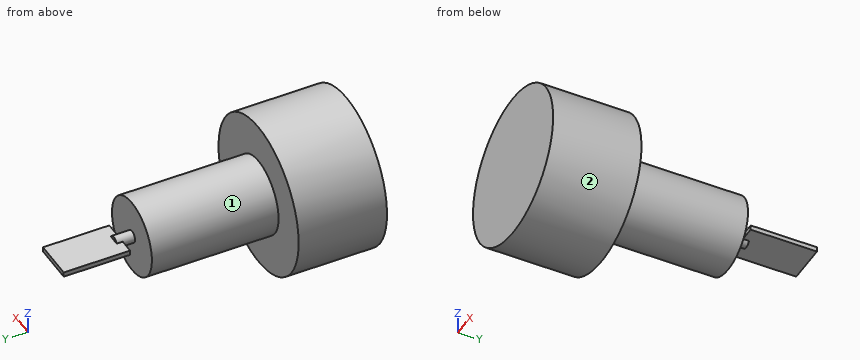
```python
from build123d import *

# Parameters (mm, degrees)
SKETCH_1_R           = 12.75
EXTRUDE_1_DEPTH      = 14.65
SKETCH_2_R           = 6.35
EXTRUDE_2_DEPTH      = 21
SKETCH_3_R           = 1
EXTRUDE_3_DEPTH      = 3
EXTRUDE_4_DEPTH      = 0.4
EXTRUDE_4_DEPTH_BACK = 0.4
SKETCH_4_W           = 6.6
SKETCH_4_H           = 11


with BuildPart() as part:
    # Sketch 1 → Extrude 1 (new body)
    with BuildSketch(Plane(origin=(0, 0, 0), x_dir=(1, 0, 0), z_dir=(0, 1, 0))):
        with Locations(Location((0, 0, 0), (0, 0, 270))):
            Circle(SKETCH_1_R)
    extrude(amount=EXTRUDE_1_DEPTH)

    # Sketch 2 → Extrude 2 (add)
    with BuildSketch(Plane(origin=(0, 14.65, 0), x_dir=(1, 0, 0), z_dir=(0, 1, 0))):
        with Locations(Location((0, 0, 0), (0, 0, 90))):
            Circle(SKETCH_2_R)
    extrude(amount=EXTRUDE_2_DEPTH)

    # Sketch 3 → Extrude 3 (add)
    with BuildSketch(Plane(origin=(0, 35.65, 0), x_dir=(1, 0, 0), z_dir=(0, 1, 0))):
        with Locations(Location((0, 0, 0), (0, 0, 270))):
            Circle(SKETCH_3_R)
    extrude(amount=EXTRUDE_3_DEPTH)

    # Sketch 4 → Extrude 4 (add, two sides: drawn at the far end of the back side and taken through both)
    with BuildSketch(Plane.XY.offset(-EXTRUDE_4_DEPTH_BACK)):
        with Locations((0.05, 43.15)):
            Rectangle(SKETCH_4_W, SKETCH_4_H)
    extrude(amount=EXTRUDE_4_DEPTH + EXTRUDE_4_DEPTH_BACK)


solid = part.part
```
The listing builds one solid part. Answer for the finished solid, in the listing's coordinates (mm). Face numbers are marked on the shaded views. A direction names the side the tool comes from. Round coordinates to 2 decimals unless told otherwise and drop trailing zeros. Loops run counter-clockwise (first coordinate to the right, second up) from the corner with the lowest first, then second, coordinate; pieces in that order, holes last.
Q1. Section C-C, the plane z = -7.25 is taken. Determine the outline of the cut face in (x, y).
Q2. Section A-A, the plane x = 0 is taken. Determine the outline of the cut face in (y, z), then the cut area to 3 significant figures.
Q3. Given pin 1 Ø10 at (x, y) = (8, 39.5) entering from -Z; pin 2 Ø4 at (x, y) = (3, 19.5) entering from -Z; pin 3 Ø8 at (x, y) = (-7, 12) entering from -Z, each flat-ended and moving along its own axis, determine where each tip first touches the part or whether it passes through.
Q4. Section B-B, the plane y = 20 is taken. Determine the outline of the cut face in (x, z), then the cut area to 3 significant figures.
Q5. Which of the six approach directions +Z, -Z, +X, -X, +Y, -Y give full straight-line access (tool end or side, diameter ignored) to the marked faces 1 and 2?
Q6. Section D-D, the plane y = 8 is taken. Determine the outline of the cut face in (x, z), then the cut area to 3 significant figures.
Q7. Find the intervals of material crossed by line 1 (Y direction, x = -4, z = -7.25); line 2 (Y direction, x = -5.25, z = -1.75); line 3 (Z direction, x = -2.75, y = 40.5), in increasing order.
Completed:
1. outline: (-10.49, 0) - (10.49, 0) - (10.49, 14.65) - (-10.49, 14.65) - close
2. outline: (0, -12.75) - (14.65, -12.75) - (14.65, -6.35) - (35.65, -6.35) - (35.65, -1) - (38.65, -1) - (38.65, -0.4) - (48.65, -0.4) - (48.65, 0.4) - (38.65, 0.4) - (38.65, 1) - (35.65, 1) - (35.65, 6.35) - (14.65, 6.35) - (14.65, 12.75) - (0, 12.75) - close
2. area: 654 mm2
3. pin 1: stops at z = -4.15
3. pin 2: stops at z = -6.27
3. pin 3: stops at z = -12.39
4. outline: circle Ø12.7 at (0, 0)
4. area: 127 mm2
5. face 1: +Y
5. face 2: +Y, -Y
6. outline: circle Ø25.5 at (0, 0)
6. area: 511 mm2
7. line 1: y = 0 to 14.65
7. line 2: y = 0 to 35.65
7. line 3: z = -0.4 to 0.4
